For this review, take the finished solid that the model builds, in its own axes (mm). Round coordinates to 2 decimals unless told otherwise and drop trailing zeros. Write each loop counter-clockwise with the first axis right and the second up, starting at its lowest first coordinate (ties: lowest second). Pieces come first, ordered by that corner, then holes. Notation, with made-up numbers: (2, 86.5) -> (49, 86.5) arc R18 ccw to (49, 121.5) -> close; hole circle Ø11 at (-9.75, 70). An arc over 180 degrees is marked (long way). Write item = value, one per line. Start each with the question number.
```python
from build123d import *

# Parameters (mm, degrees)
FILLET1_R = 1.27


with BuildPart() as part:
    # Sketch1 → Revolve1 (revolve)
    with BuildSketch(Plane(origin=(0, 0, 0), x_dir=(0, 0, -1), z_dir=(1, 0, 0))):
        with BuildLine():
            Line((0, 27.94), (0, 32.385))
            Line((0, 32.385), (25.4, 32.385))
            Line((25.4, 32.385), (25.4, 27.94))
            ThreePointArc((25.4, 27.94), (25.028025612, 28.838025612), (24.13, 29.21))
            Line((24.13, 29.21), (1.27, 29.21))
            ThreePointArc((1.27, 29.21), (0.371974388, 28.838025612), (0, 27.94))
        make_face()
    revolve(axis=Axis((0, 0, 0), (0, 0, -1)))

    # Fillet1
    fillet1_edges = [part.edges().sort_by_distance(p)[0] for p in [
        (0, -32.385, -25.4),
        (0, -32.385, 0),
    ]]
    fillet(fillet1_edges, radius=FILLET1_R)


solid = part.part
```
1. Wall thickness on L1, parallel to X at y = 0, z = -15.75 (3 decimals); L2, parallel to X at y = 17, z = -8.75; L3, parallel to Y at x = 10.5, z = -19.25: over which ranges is each line inside the solid? List them lowest first. Write a range as from..to.
2. Draft analysis for pull direction X (two halves, no side actions). For faces 1 (the cylindrical face through (-19.706, -25.7, -12.86)), 2 (the cylindrical face through (19.74, -21.53, -12.54)), state which applies: +X half, -X half, draft (parallel to the pull), parting line (faces both ways), or undercut.
3. Consider section A-A, the plane y = 0. Give the boundary of the cut face in (x, z) (3 decimals).
4. Consider section C-C, the plane z = -12. Give the boundary of the cut face in (x, y) (3 decimals), then the cut area to 3 significant figures.
5. Clearance check with flat-ended pins moving along their axes: pin 1 Ø1 at (x, y) = (19, 18) entering from -Z; pin 2 Ø4 at (x, z) = (-6, -20) entering from -Y; pin 3 Ø5 at (y, z) = (2, -16.5) entering from -X (3 decimals); pin 4 Ø8 at (x, z) = (24.5, -4) entering from +Y. State where each tip first meets the part, or that it passes through.
Outcome:
q1.L1 = -32.385..-29.21, 29.21..32.385
q1.L2 = -27.56..-23.75, 23.75..27.56
q1.L3 = -30.64..-27.26, 27.26..30.64
q2.face_1 = parting line
q2.face_2 = undercut
q3.outline = (-32.385, -24.13) arc R1.27 ccw to (-31.115, -25.4) -> (-27.94, -25.4) arc R1.27 cw to (-29.21, -24.13) -> (-29.21, -1.27) arc R1.27 cw to (-27.94, 0) -> (-31.115, 0) arc R1.27 ccw to (-32.385, -1.27) -> close; (27.94, -25.4) -> (31.115, -25.4) arc R1.27 ccw to (32.385, -24.13) -> (32.385, -1.27) arc R1.27 ccw to (31.115, 0) -> (27.94, 0) arc R1.27 cw to (29.21, -1.27) -> (29.21, -24.13) arc R1.27 cw to start
q4.outline = circle Ø64.77 at (0, 0); hole circle Ø58.42 at (0, 0)
q4.area = 614 mm2
q5.pin_1 = through
q5.pin_2 = -32.14
q5.pin_3 = -32.385
q5.pin_4 = 25.07
